Drawing for the job (mm, zero at the part's lowest x, y, z). A direction names the side the tool comes from. Coordinates: 2 decimals unless noted, no trailing zeros. Write each loop counter-clockwise with the first axis right and the second up, starting at its lowest first coordinate (ties: lowest second). Pieces come first, ordered by that corner, then holes. Notation, with made-up numbers: M 26,0.25 L 43,0.25 A36 cw 43,39.25 Z; hole C 26.25,-4 d5. An arc over 180 degrees is marked long. Use a Markdown table: item, result. Add a question column.
Q1. Pin check, flat tips, straight feed: pin 1 Ø4 at (x, y) = (6, 9.5) entering from -Z; pin 2 Ø2 at (y, z) = (8, 15) entering from +X; pin 3 Ø3.5 at (x, z) = (16.25, 23.75) entering from +Y; pin 4 Ø2 at (x, y) = (27, 12) entering from -Z. Stop position of each tip, or through.
Q2. Mould opens along Z. For the marked faces 1, 2 and 3 say: released by +Z, released by -Z, zero draft, split by the parting line, or undercut.
Q3. Slice it at B-B on z = 23.75. Write the cut outline in (x, y), then the cut area to 3 significant figures.
Q4. Slice it at A-A on x = 16.25. Write the cut outline in (y, z), then the cut area to 3 significant figures.
Q5. Slice it at C-C on y = 8.5. Write the cut outline in (x, z), then the cut area to 3 significant figures.
Q6. Tool access for the marked faces 4 and 5: list every direction of +Z, -Z, +X, -X, +Y, -Y with a clear straight run to the whole face (end or side of a thin tool).
Q7. Wall check: L1, parallel to Z at x = 18, y = 3.25; L2, parallel to Z at x = 15, y = 13.25; L3, parallel to X at y = 10.25, z = 8.75. Give the ranges that are in metal, low to high. Write a range as from..to.
Q8. Slice it at D-D on x = 2.5. Write the cut outline in (y, z).
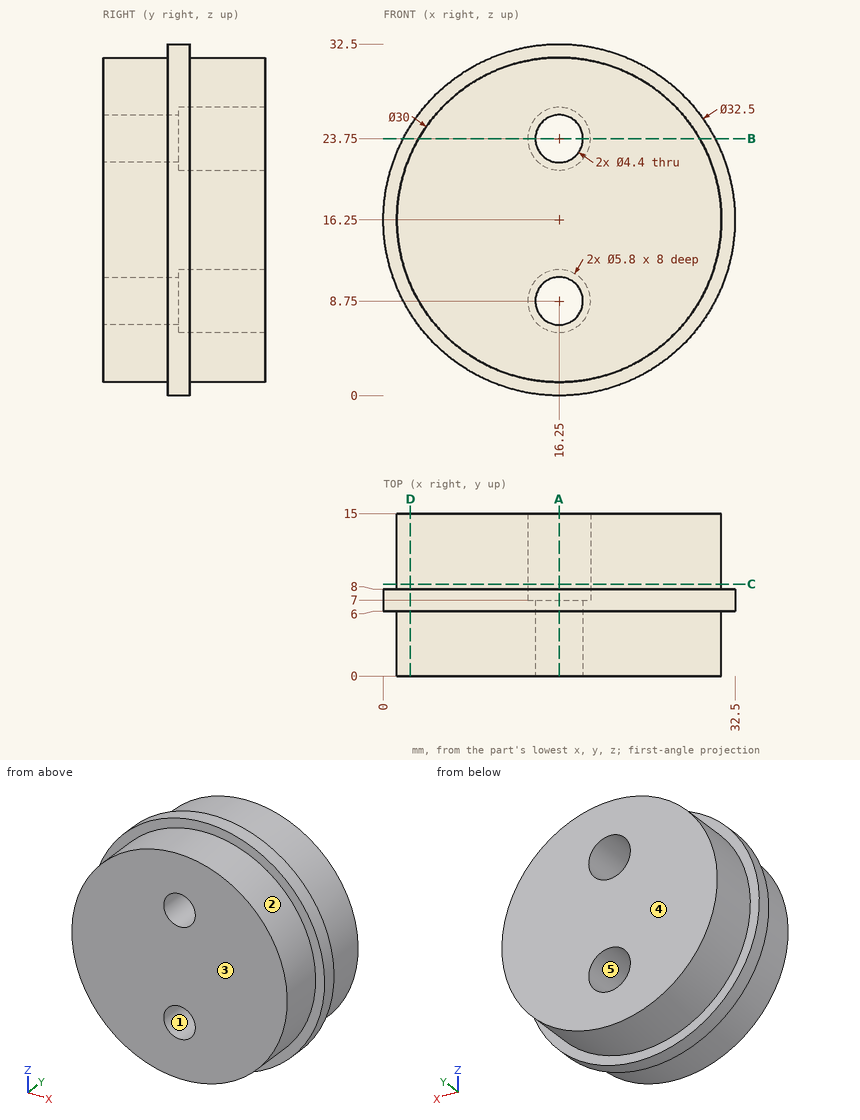
Recorded:
| question | item | result |
|---|---|---|
| 1 | pin 1 | z = 2.67 |
| 1 | pin 2 | x = 32.5 |
| 1 | pin 3 | through |
| 1 | pin 4 | z = 4.85 |
| 2 | face 1 | undercut |
| 2 | face 2 | split by the parting line |
| 2 | face 3 | zero draft |
| 3 | outline | M 1.83,6 L 3.26,6 L 3.26,0 L 14.05,0 L 14.05,7 L 13.35,7 L 13.35,15 L 3.26,15 L 3.26,8 L 1.83,8 Z; M 18.45,0 L 29.24,0 L 29.24,6 L 30.67,6 L 30.67,8 L 29.24,8 L 29.24,15 L 19.15,15 L 19.15,7 L 18.45,7 Z |
| 3 | area | 318 mm² |
| 4 | outline | M 0,1.25 L 6,1.25 L 6,0 L 8,0 L 8,1.25 L 15,1.25 L 15,5.85 L 7,5.85 L 7,6.55 L 0,6.55 Z; M 0,10.95 L 7,10.95 L 7,11.65 L 15,11.65 L 15,20.85 L 7,20.85 L 7,21.55 L 0,21.55 Z; M 0,25.95 L 7,25.95 L 7,26.65 L 15,26.65 L 15,31.25 L 8,31.25 L 8,32.5 L 6,32.5 L 6,31.25 L 0,31.25 Z |
| 4 | area | 301 mm² |
| 5 | outline | C 16.25,16.25 d30; hole C 16.25,8.75 d5.8; hole C 16.25,23.75 d5.8 |
| 5 | area | 654 mm² |
| 6 | face 4 | +Z, -Z, +X, -X, +Y |
| 6 | face 5 | +Y |
| 7 | L1 | 1.35..7.42, 10.08..22.42, 25.08..31.15 |
| 7 | L2 | 1.3..6.13, 11.37..21.13, 26.37..31.2 |
| 7 | L3 | 3.26..13.35, 19.15..29.24 |
| 8 | outline | M 0,10.26 L 6,10.26 L 6,7.59 L 8,7.59 L 8,10.26 L 15,10.26 L 15,22.24 L 8,22.24 L 8,24.91 L 6,24.91 L 6,22.24 L 0,22.24 Z |
